from build123d import *

# Parameters (mm, degrees)
F1_DEPTH = 101.6
F2_DEPTH = 50.8
F3_DEPTH = 25.4


with BuildPart() as f1:
    # F0 (on Front) → F1 (new body)
    with BuildSketch(Plane.XZ):
        with BuildLine():
            add(Edge.make_bspline(
                [(63.5, 101.6), (32.3093875408, 101.6), (13.2439655959, 62.1035214404)],
                knots=[3.1415926536, 3.1415926536, 3.1415926536, 4.0547434617, 4.0547434617, 4.0547434617], degree=2, weights=[1, 0.8975675831, 1]))
            ThreePointArc((13.2439655959, 62.1035214404), (49.3621404284, 39.9453262889), (63.5, 0))
            Line((63.5, 0), (63.5, 101.6))
        make_face()
        with BuildLine():
            ThreePointArc((63.5, 0), (49.3621404284, 39.9453262889), (13.2439655959, 62.1035214404))
            add(Edge.make_bspline(
                [(13.2439655959, 62.1035214404), (0, 34.6669399309), (0, 0)],
                knots=[4.0547434617, 4.0547434617, 4.0547434617, 4.7123889804, 4.7123889804, 4.7123889804], degree=2, weights=[1, 0.9464231645, 1]))
            add(Edge.make_bspline(
                [(0, 0), (0, -34.6669399309), (13.2439655959, -62.1035214404)],
                knots=[4.7123889804, 4.7123889804, 4.7123889804, 5.370034499, 5.370034499, 5.370034499], degree=2, weights=[1, 0.9464231645, 1]))
            ThreePointArc((13.2439655959, -62.1035214404), (49.3621404284, -39.9453262889), (63.5, 0))
        make_face()
    extrude(amount=F1_DEPTH)

    # F0 (on Front) → F2 (join)
    with BuildSketch(Plane.XZ):
        with BuildLine():
            ThreePointArc((-51.59375, 37.0180356169), (-37.0237934934, 21.0006510316), (-31.75, 0))
            ThreePointArc((-31.75, 0), (-37.0237934934, -21.0006510316), (-51.59375, -37.0180356169))
            ThreePointArc((-51.59375, -37.0180356169), (-22.9128106244, -59.2220660674), (13.2439655959, -62.1035214404))
            add(Edge.make_bspline(
                [(0, 0), (0, -34.6669399309), (13.2439655959, -62.1035214404)],
                knots=[4.7123889804, 4.7123889804, 4.7123889804, 5.370034499, 5.370034499, 5.370034499], degree=2, weights=[1, 0.9464231645, 1]))
            add(Edge.make_bspline(
                [(13.2439655959, 62.1035214404), (0, 34.6669399309), (0, 0)],
                knots=[4.0547434617, 4.0547434617, 4.0547434617, 4.7123889804, 4.7123889804, 4.7123889804], degree=2, weights=[1, 0.9464231645, 1]))
            ThreePointArc((13.2439655959, 62.1035214404), (-22.9128106244, 59.2220660674), (-51.59375, 37.0180356169))
        make_face()
        with BuildLine():
            ThreePointArc((-51.59375, -37.0180356169), (-37.0237934934, -21.0006510316), (-31.75, 0))
            ThreePointArc((-31.75, 0), (-37.0237934934, 21.0006510316), (-51.59375, 37.0180356169))
            ThreePointArc((-51.59375, 37.0180356169), (-63.5, 0), (-51.59375, -37.0180356169))
        make_face()
    extrude(amount=F2_DEPTH)

    # F0 (on Front) → F3 (join)
    with BuildSketch(Plane.XZ):
        with BuildLine():
            ThreePointArc((-51.59375, -37.0180356169), (-63.5, 0), (-51.59375, 37.0180356169))
            ThreePointArc((-51.59375, 37.0180356169), (-120.65, 0), (-51.59375, -37.0180356169))
        make_face()
    extrude(amount=F3_DEPTH)


solid = f1.part
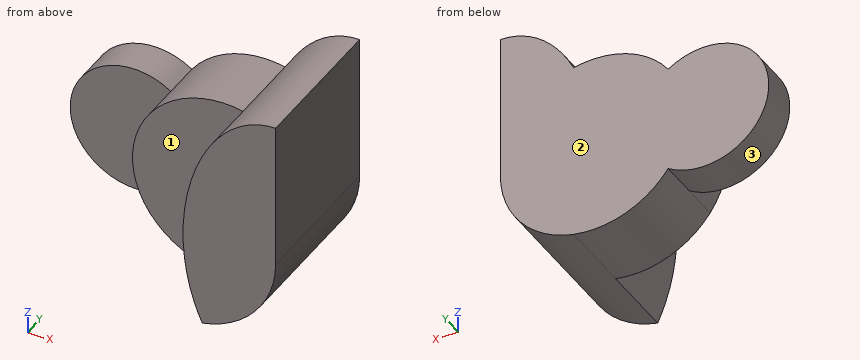
Geometry: final body of the model. Coordinates: model frame, mm. Face numbers are marked on the shaded views. Give positions to 0.01 mm unless a question says otherwise; leave off trailing zeros. Write each loop counter-clockwise with the first axis right and the second up, starting at its lowest first coordinate (ties: lowest second). Pieces come first, ordered by that corner, then holes. Notation, with made-up numbers: (46.5, -25.5) - (94.5, -25.5) arc R21 ccw to (94.5, -12.5) - close; hole circle Ø11 at (29, -15). An arc over 180 degrees is marked (long way). Return JSON: item names as keys, results as strings. Group by question number.
1) Line query: line 1 (Y direction, x = -41.5, z = -16.5); line 2 (X direction, y = -93.5, z = 2); line 3 (X direction, y = -70, z = -19.5). Output: solid intervals per line, ascending.
2) Section A-A on x = -76.2. Return the cut outline in (y, z), plus the area to 3 significant figures.
3) First-contact query: P1, Ø10, axis at x = 39, y = -18.5, coming from the -Z side; P2, Ø2, axis at y = -71, z = 73, coming from the -X side; P3, Ø23, axis at x = -27, z = 28.5, coming from the -Y side. Flat tips, straight axial feed; report the tip coordinate or a pass-through.
4) Mould query, pull axis Y, two halves, no side actions, for the marked faces 1, 2 and 3. Classes: released by +Y, released by -Y, zero draft, split by the parting line, or undercut.
5) Section B-B on x = -99.5. Return the cut outline in (y, z), plus the area to 3 significant figures.
Filled in:
{
 "1": {"line 1": "y = -50.8 to 0", "line 2": "x = 0.01 to 63.5", "line 3": "x = 1.18 to 60.43"},
 "2": {"outline": "(-25.4, -44.45) - (0, -44.45) - (0, 44.45) - (-25.4, 44.45) - close", "area": "2,260 mm^2"},
 "3": {"P1": "stops at z = -53.63", "P2": "stops at x = 18.7", "P3": "stops at y = -50.8"},
 "4": {"face 1": "released by -Y", "face 2": "released by +Y", "face 3": "zero draft"},
 "5": {"outline": "(-25.4, -37.85) - (0, -37.85) - (0, 37.85) - (-25.4, 37.85) - close", "area": "1,920 mm^2"}
}
